The figure shows three views and two pictorial views of one solid part (mm, origin at its lowest corner). Answer the questions. A direction names the side the tool comes from. Coordinates: 2 decimals unless noted, no trailing zeros. Order: outer loops, then holes, each group sorted by start corner. A loop starts at its lowest first (then second) coordinate and runs counter-clockwise, first axis right, second up. Notation, with made-up numbers: (30.25, -38) - (72.25, -38) arc R27 cw to (72.25, -17) - close; hole circle Ø5 at (82.25, 46.25). An arc over 180 degrees is marked (long way). Use one line per item in the form item = value. Start each with the question number.
Item 1: Section A-A, the plane z = 127 is taken. Count the separate pieces of the cut face and the enclosed holes in it, and give its area (3 significant figures).
Item 2: Section B-B, the plane y = 254 is taken. Write down the section's boundary in (x, z).
Item 3: Section D-D, the plane z = 299 is taken. Write down the section's boundary in (x, y).
Item 4: The mould has two halves that part along Y. Classify the marked faces 1, 2 and 3: released by +Y, released by -Y, zero draft, split by the parting line, or undercut.
Item 5: Section C-C, the plane x = 678 is taken. Write down the section's boundary in (y, z).
Item 6: A tool of negligible diameter and unlimited length cuts with its end or side. For the marked faces 4 and 5, from which of +Z, -Z, +X, -X, +Y, -Y can it reach the whole face along a straight path? Write none if from no direction.
Item 7: Consider line 1 along Z through (x, y) = (1009, 254); line 2 along Y through (x, z) = (383, 235.5); line 3 along X through (y, z) = (1176.5, 260.5). Determine where each line is inside the solid, lowest interval first. Write a range as [from, to].
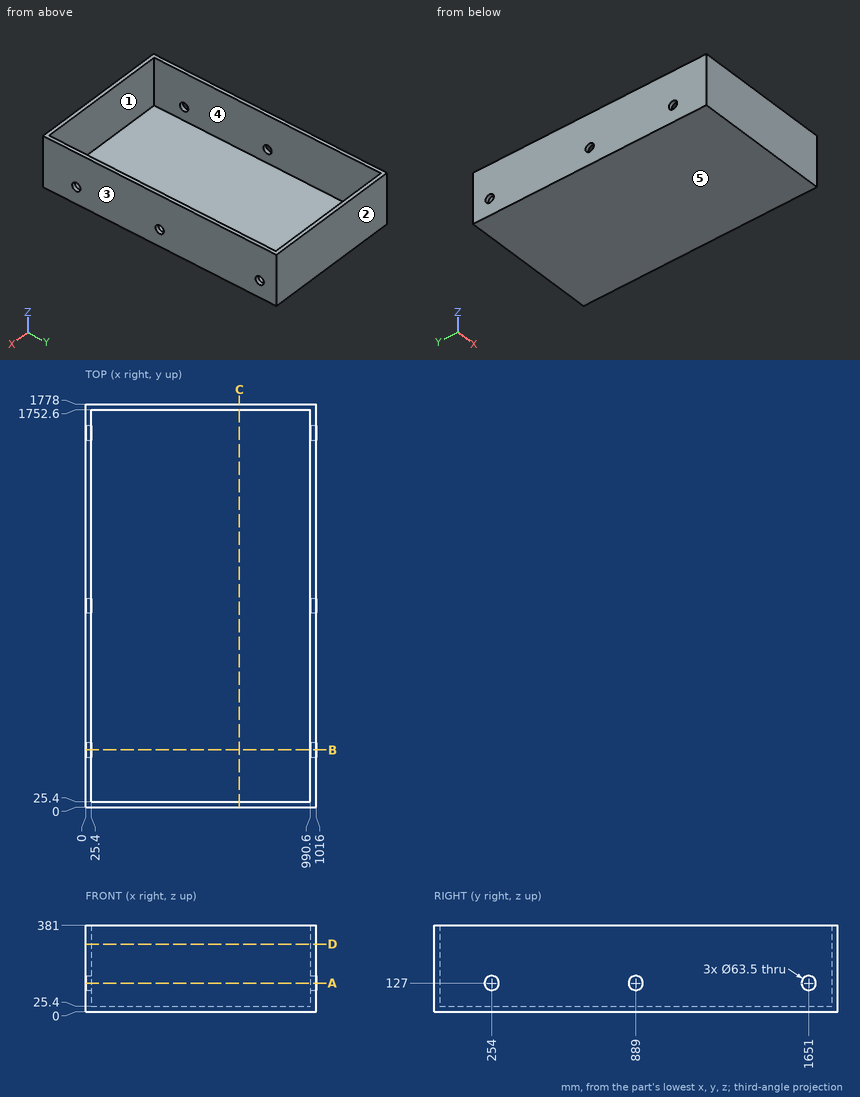
Response:
q1.separate_pieces = 6
q1.enclosed_holes = 0
q1.area = 130,000 mm2
q2.outline = (0, 0) - (1016, 0) - (1016, 95.25) - (990.6, 95.25) - (990.6, 25.4) - (25.4, 25.4) - (25.4, 95.25) - (0, 95.25) - close; (0, 158.75) - (25.4, 158.75) - (25.4, 381) - (0, 381) - close; (990.6, 158.75) - (1016, 158.75) - (1016, 381) - (990.6, 381) - close
q3.outline = (0, 0) - (1016, 0) - (1016, 1778) - (0, 1778) - close; hole (25.4, 25.4) - (990.6, 25.4) - (990.6, 1752.6) - (25.4, 1752.6) - close
q4.face_1 = undercut
q4.face_2 = released by +Y
q4.face_3 = zero draft
q5.outline = (0, 0) - (1778, 0) - (1778, 381) - (1752.6, 381) - (1752.6, 25.4) - (25.4, 25.4) - (25.4, 381) - (0, 381) - close
q6.face_4 = +Z
q6.face_5 = -Z, +X, -X, +Y, -Y
q7.line_1 = [0, 95.25], [158.75, 381]
q7.line_2 = [0, 25.4], [1752.6, 1778]
q7.line_3 = [0, 25.4], [990.6, 1016]
